Check sheet for the modelled part. Datum: model origin and axes. Units: mm. Coordinates: 2 decimals unless noted, no trailing zeros. Write each loop counter-clockwise with the first axis right and the second up, starting at its lowest first coordinate (ties: lowest second). Pieces come first, ordered by that corner, then holes. Notation, with made-up numbers: (-34.75, 23.25) - (13.25, 23.25) arc R27 ccw to (13.25, 61.25) - close; hole circle Ø6 at (46, 12). An arc over 180 degrees is marked (long way). Use one line per item in the form item = value. Start each with the question number.
1. Scan lines: line 1 along Y through (x, z) = (0.3, 3); line 2 along Z through (x, y) = (0.15, 8); line 3 along Y through (x, z) = (0.45, -7.25). Record each from-to range of solid material in increasing order.
2. Go/stop test with a flat-tipped pin: pin 1 Ø10 at (y, z) = (7.5, 1) entering from -X. Record where the tip stops, or that it passes through.
3. Cross-section at A-A on x = 0.2. Record the boundary of the cut face in (y, z), then the cut area to 3 significant figures.
```python
from build123d import *

# Parameters (mm, degrees)
RESSALTO_EXTRUS_O1_DEPTH = 0.5
FILETE2_R                = 0.12
ESBO_O3_R                = 0.35
CORTE_EXTRUS_O1_DEPTH    = 0.5


with BuildPart() as part:
    # Esboço1 → Ressalto-extrusão1 (new body)
    with BuildSketch(Plane(origin=(0, 0, 0), x_dir=(0, 0, -1), z_dir=(1, 0, 0))):
        with BuildLine():
            Line((7.755818376, -6.312470303), (7.546549647, -5.770579557))
            ThreePointArc((7.546549647, -5.770579557), (8.951430844, -3.181491135), (9.495678331, -0.286518819))
            Line((9.495678331, -0.286518819), (10, 0))
            Line((10, 0), (9.495513044, 0.291945241))
            ThreePointArc((9.495513044, 0.291945241), (8.903037488, 3.314501996), (7.374694694, 5.988645771))
            Line((7.374694694, 5.988645771), (7.564299357, 6.540747299))
            Line((7.564299357, 6.540747299), (6.979531804, 6.444853435))
            ThreePointArc((6.979531804, 6.444853435), (3.95093379, 8.639451498), (0.30994469, 9.494942564))
            Line((0.30994469, 9.494942564), (0, 10))
            Line((0, 10), (-0.312056411, 9.494873395))
            ThreePointArc((-0.312056411, 9.494873395), (-4.079212885, 8.579628328), (-7.167066673, 6.235635918))
            Line((-7.167066673, 6.235635918), (-7.755818376, 6.312470303))
            Line((-7.755818376, 6.312470303), (-7.545539803, 5.771899955))
            ThreePointArc((-7.545539803, 5.771899955), (-8.951152463, 3.182274278), (-9.495678331, 0.286518819))
            Line((-9.495678331, 0.286518819), (-10, 0))
            Line((-10, 0), (-9.495513044, -0.291945241))
            ThreePointArc((-9.495513044, -0.291945241), (-8.902746815, -3.315282665), (-7.373644327, -5.98993901))
            Line((-7.373644327, -5.98993901), (-7.564299357, -6.540747299))
            Line((-7.564299357, -6.540747299), (-6.976885209, -6.447718417))
            ThreePointArc((-6.976885209, -6.447718417), (-3.949160195, -8.640262366), (-0.30994469, -9.494942564))
            Line((-0.30994469, -9.494942564), (0, -10))
            Line((0, -10), (0.312056411, -9.494873395))
            ThreePointArc((0.312056411, -9.494873395), (4.077471711, -8.580455958), (7.16453525, -6.238544273))
            Line((7.16453525, -6.238544273), (7.755818376, -6.312470303))
        make_face()
    extrude(amount=RESSALTO_EXTRUS_O1_DEPTH)

    # Filete2
    filete2_edges = [part.edges().sort_by_distance(p)[0] for p in [
        (0.5, -0.14325941, -9.747839166),
        (0.5, 0.145972621, -9.747756522),
        (0.5, 3.314501996, -8.903037488),
        (0.5, 6.264696535, -7.469497026),
        (0.5, 6.492800367, -7.271915581),
        (0.5, 8.639451498, -3.95093379),
        (0.5, 9.747471282, -0.154972345),
        (0.5, 9.747436698, 0.156028205),
        (0.5, 8.579628328, 4.079212885),
        (0.5, 6.274053111, 7.461442524),
        (0.5, -6.04152493, -7.651184011),
        (0.5, 6.042185129, 7.650679089),
        (0.5, 3.182274278, 8.951152463),
        (0.5, 0.14325941, 9.747839166),
        (0.5, -0.145972621, 9.747756522),
        (0.5, -3.315282665, 8.902746815),
        (0.5, -6.265343155, 7.468971842),
        (0.5, -6.494232858, 7.270592283),
        (0.5, -8.640262366, 3.949160195),
        (0.5, -9.747471282, 0.154972345),
        (0.5, -3.181491135, -8.951430844),
        (0.5, -9.747436698, -0.156028205),
        (0.5, -8.580455958, -4.077471711),
        (0.5, -6.275507288, -7.460176813),
    ]]
    fillet(filete2_edges, radius=FILETE2_R)

    # Esboço3 → Corte-extrusão1 (cut)
    with BuildSketch(Plane(origin=(0.5, 0, 0), x_dir=(0, 0, -1), z_dir=(1, 0, 0))):
        with Locations((3.249745018, 7.105782814)):
            Circle(ESBO_O3_R)
        with Locations((-3.225311319, -7.056999805)):
            Circle(ESBO_O3_R)
    extrude(amount=-CORTE_EXTRUS_O1_DEPTH, mode=Mode.SUBTRACT)


solid = part.part
```
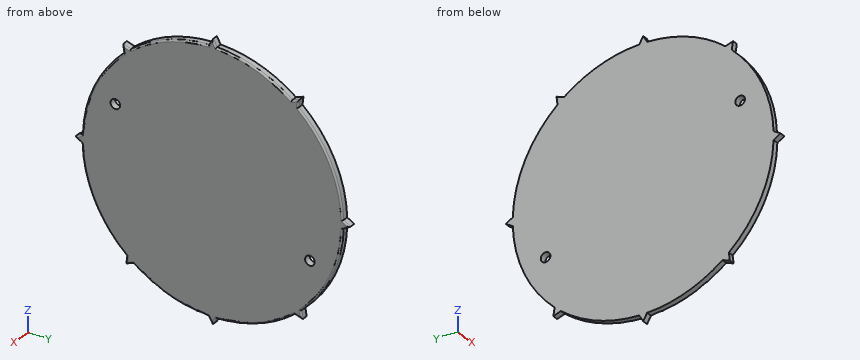
Final values:
q1.line_1 = -9.01 to -7.32, -6.79 to 9.01
q1.line_2 = -5.12 to 5.12
q1.line_3 = -6.23 to 6.47
q2.pin_1 = 0
q3.outline = (-10, 0) - (-9.49, -0.31) arc R9.5 ccw to (-6.24, -7.16) - (-6.31, -7.76) - (-5.77, -7.55) arc R9.5 ccw to (-0.29, -9.5) - (0, -10) - (0.29, -9.5) arc R9.5 ccw to (5.99, -7.37) - (6.54, -7.56) - (6.44, -6.98) arc R9.5 ccw to (9.49, -0.31) - (10, 0) - (9.49, 0.31) arc R9.5 ccw to (6.24, 7.17) - (6.31, 7.76) - (5.77, 7.55) arc R9.5 ccw to (0.29, 9.5) - (0, 10) - (-0.29, 9.5) arc R9.5 ccw to (-5.99, 7.37) - (-6.54, 7.56) - (-6.45, 6.98) arc R9.5 ccw to (-9.49, 0.31) - close; hole circle Ø0.7 at (-7.06, 3.23); hole circle Ø0.7 at (7.11, -3.25)
q3.area = 284 mm²
